```python
from build123d import *

# Parameters (mm, degrees)
F0_W      = 30
F0_H      = 28
F1_DEPTH  = 11
F2_R      = 5
F3_W      = 30
F3_H      = 5.535902
F4_DEPTH  = 15
F5_R      = 1.6
F6_DEPTH  = 16
F7_W      = 30
F7_H      = 4.997426
F8_DEPTH  = 4
F9_W      = 30
F9_H      = 2.822344
F10_DEPTH = 15
F12_DEPTH = 3


with BuildPart() as f1:
    # F0 (on Top) → F1 (new body)
    with BuildSketch(Plane.XY):
        Rectangle(F0_W, F0_H)
    extrude(amount=F1_DEPTH)

    # F2
    f2_edges = [f1.edges().sort_by_distance(p)[0] for p in [
        (15, 14, 5.5),
        (-15, 14, 5.5),
    ]]
    fillet(f2_edges, radius=F2_R)

    # F3 (on face) → F4 (join)
    with BuildSketch(Plane(origin=(0, 0, 0), x_dir=(1, 0, 0), z_dir=(0, 0, -1))):
        with Locations((0, 11.232049)):
            Rectangle(F3_W, F3_H)
    extrude(amount=F4_DEPTH)

    # F5 (on face) → F6 (cut)
    with BuildSketch(Plane(origin=(0, -8.464098, 0), x_dir=(-1, 0, 0), z_dir=(0, 1, 0))):
        with Locations((-6.3, -8.5)):
            Circle(F5_R)
        with Locations((8.1, -8.6)):
            Circle(F5_R)
    extrude(amount=-F6_DEPTH, mode=Mode.SUBTRACT)

    # F7 (on face) → F8 (join)
    with BuildSketch(Plane.XY.offset(11)):
        with Locations((0, -11.501287)):
            Rectangle(F7_W, F7_H)
    extrude(amount=F8_DEPTH)

    # F9 (on face) → F10 (join)
    with BuildSketch(Plane(origin=(0, -9.002574, 0), x_dir=(-1, 0, 0), z_dir=(0, 1, 0))):
        with Locations((0, 13.588828)):
            Rectangle(F9_W, F9_H)
    extrude(amount=F10_DEPTH)

    # F11 (on face) → F12 (cut)
    with BuildSketch(Plane.XY.offset(15)):
        with BuildLine():
            Line((-5.1, 5.647501), (-5.1, -0.052499))
            ThreePointArc((-5.1, -0.052499), (-5.6e-05, -5.128539), (5.099887, -0.052499))
            Line((5.099887, -0.052499), (5.099887, 5.647501))
            Line((5.099887, 5.647501), (5.099887, 5.997426))
            Line((5.099887, 5.997426), (-5.1, 5.997426))
            Line((-5.1, 5.997426), (-5.1, 5.647501))
        make_face()
    extrude(amount=-F12_DEPTH, mode=Mode.SUBTRACT)


solid = f1.part
```
Work out the finished part from the listing and answer in its coordinate system (mm). A direction names the side the tool comes from. Coordinates: 2 decimals unless noted, no trailing zeros. Loops run counter-clockwise (first coordinate to the right, second up) from the corner with the lowest first, then second, coordinate; pieces in that order, holes last. Notation, with made-up numbers: (5.25, 3) -> (37.25, 3) arc R26 ccw to (37.25, 37) -> close; hole circle Ø6 at (61, -37). An arc over 180 degrees is marked (long way). Answer as CSV lines item,"result".
Q1. Find the intervals of material crossed by probe 1 along Z at (x, y) = (-8.1, -12.5); probe 2 along Z at (x, y) = (6.3, -10.95); probe 3 along Y at (x, z) = (-7.5, -4.75), in increasing order.
Findings:
probe 1,"z = -15 to -10.2, -7 to 15"
probe 2,"z = -15 to -10.1, -6.9 to 15"
probe 3,"y = -14 to -8.46"
Q2. A tool of negligible diameter and unlimited length cuts with its end or side. For faces 5 (the face through (-10, 5.997, 14)), 6 (the face through (0, 14, 5)), 7 (the face through (0, 3, 0)), 8 (the face through (0, -9.003, 12)), from which of +Z, -Z, +X, -X, +Y, -Y can it reach the whole face along a straight path? Write none if from no direction.
Findings:
face 5,"+Z, +X, -X, +Y"
face 6,"+Z, -Z, +X, -X, +Y"
face 7,"-Z, +X, -X, +Y"
face 8,"+X, -X, +Y"
Q3. The part is cut by section C-C on y = -9.5. Write down the section's boundary in (x, z).
Findings:
outline,"(-15, -15) -> (15, -15) -> (15, 15) -> (-15, 15) -> close; hole circle Ø3.2 at (-8.1, -8.6); hole circle Ø3.2 at (6.3, -8.5)"
Q4. Each of these flat-tipped pins is pushed along its axis until it touches: pin 1 (2.5 mm diameter, centred on x = -10, z = 13, fed in from +Y); pin 2 (1.5 mm diameter, centred on x = -1, y = 8, fed in from +Z); pin 3 (3.5 mm diameter, centred on x = 6.3, z = -8.5, fed in from +Y); pin 4 (16.5 mm diameter, centred on x = 3.5, y = -1.5, fed in from -Z). Where does it stop, or does it pass through?
Findings:
pin 1,"stops at y = 6"
pin 2,"stops at z = 11"
pin 3,"stops at y = -8.46"
pin 4,"stops at z = -15"
Q5. The part is cut by section A-A on y = -6.25. Write down the section's boundary in (x, z).
Findings:
outline,"(-15, 0) -> (15, 0) -> (15, 11) -> (-15, 11) -> close; (-15, 12.18) -> (15, 12.18) -> (15, 15) -> (-15, 15) -> close"
Q6. The part is cut by section D-D on x = 3. Write down the section's boundary in (y, z), and give its area (3 significant figures).
Findings:
outline,"(-14, -15) -> (-8.46, -15) -> (-8.46, 0) -> (14, 0) -> (14, 11) -> (-9, 11) -> (-9, 12.18) -> (-4.15, 12.18) -> (-4.15, 15) -> (-14, 15) -> close"
area,"425 mm²"
Q7. The part is cut by section B-B on x = 6.3. Write down the section's boundary in (y, z), and give its area (3 significant figures).
Findings:
outline,"(-14, -15) -> (-8.46, -15) -> (-8.46, -10.1) -> (-14, -10.1) -> close; (-14, -6.9) -> (-8.46, -6.9) -> (-8.46, 0) -> (14, 0) -> (14, 11) -> (-9, 11) -> (-9, 12.18) -> (6, 12.18) -> (6, 15) -> (-14, 15) -> close"
area,"436 mm²"
Q8. For a pull along X with two mould halves and no side action, classify faces 1 (the face through (-0.112, -5.127, 13.609)), 2 (the face through (-5.1, 3, 14)), 3 (the face through (4, -5, 12.178)), 4 (the face through (15, -5, 3)) as +X half, -X half, draft (parallel to the pull), parting line (faces both ways), or undercut.
Findings:
face 1,"undercut"
face 2,"undercut"
face 3,"draft"
face 4,"+X half"
